Model file for the job. Use its own axes, mm. Coordinates: 2 decimals unless noted, no trailing zeros. Write each loop counter-clockwise with the first axis right and the second up, starting at its lowest first coordinate (ties: lowest second). Pieces come first, ordered by that corner, then holes. Notation, with made-up numbers: (80.25, 79.25) -> (105.25, 79.25) arc R5 ccw to (105.25, 86.25) -> close; hole circle Ø8 at (84.25, 23). An arc over 180 degrees is marked (long way). Write item = value, one per line. Start each with the question number.
from build123d import *

# Parameters (mm, degrees)
SKETCH1_R           = 17
BOSS_EXTRUDE2_DEPTH = 8
CHAMFER1_SIZE       = 1


with BuildPart() as part:
    # Sketch1 → Boss-Extrude2 (new body)
    with BuildSketch(Plane.XY):
        Circle(SKETCH1_R)
    extrude(amount=BOSS_EXTRUDE2_DEPTH)

    # Sketch3 → Cut-Revolve2 (revolve, cut)
    with BuildSketch(Plane(origin=(0, 0, 0), x_dir=(1, 0, 0), z_dir=(0, 1, 0)), mode=Mode.PRIVATE) as cut_revolve2_sk:
        Polygon((0, 0), (0, -8), (6, -8), (6, -6), (12, 0), align=None)
    revolve(cut_revolve2_sk.sketch.rotate(Axis((0, 0, 0), (0, 0, 1)), 180), axis=Axis((0, 0, 0), (0, 0, 1)), mode=Mode.SUBTRACT)

    # Chamfer1
    chamfer1_edges = [part.edges().sort_by_distance(p)[0] for p in [
        (-17, 0, 0),
        (-17, 0, 8),
    ]]
    chamfer(chamfer1_edges, length=CHAMFER1_SIZE)


solid = part.part
(1) Mould opens along X. For faces 1 (the face through (2, 12, 0)), 2 (the face through (9.139, 14.334, 3.958)), 3 (the face through (-5.723, -1.802, 6.986)) say: released by +X, released by -X, zero draft, split by the parting line, or undercut.
(2) Saw through at A-A (x = 0). Give the cut face in (y, z), then the cut area to 3 significant figures.
(3) Drill centre lines: line 1 along Y through (x, z) = (0, 6.5); line 2 along Y through (x, z) = (0, 7.35); line 3 along X through (y, z) = (8, 3). Where is each one in solid material? Low to high.
(4) Drop flat-ended pins along their axis: pin 1 Ø3 at (y, z) = (2.5, 6.5) entering from -X; pin 2 Ø1 at (x, y) = (6, 5) entering from -Z; pin 3 Ø1.5 at (y, z) = (6.5, 1.5) entering from -X; pin 4 Ø7 at (x, y) = (0, 0) entering from -Z. Give the stop position or say it passes through.
(5) Saw through at D-D (z = 4.5). Give the cut face in (x, y), then the cut area to 3 significant figures.
(6) Saw through at C-C (z = 0.5). Give the cut face in (x, y).
Returned:
q1.face_1 = zero draft
q1.face_2 = split by the parting line
q1.face_3 = undercut
q2.outline = (-17, 1) -> (-16, 0) -> (-12, 0) -> (-6, 6) -> (-6, 8) -> (-16, 8) -> (-17, 7) -> close; (6, 6) -> (12, 0) -> (16, 0) -> (17, 1) -> (17, 7) -> (16, 8) -> (6, 8) -> close
q2.area = 138 mm2
q3.line_1 = -17 to -6, 6 to 17
q3.line_2 = -16.65 to -6, 6 to 16.65
q3.line_3 = -15 to -4.12, 4.12 to 15
q4.pin_1 = -16.97
q4.pin_2 = 3.69
q4.pin_3 = -16
q4.pin_4 = through
q5.outline = circle Ø34 at (0, 0); hole circle Ø15 at (0, 0)
q5.area = 731 mm2
q6.outline = circle Ø33 at (0, 0); hole circle Ø23 at (0, 0)
